Source: CAD feature listing. Evaluate the final solid. Frame: model axes, mm. Coordinates: 2 decimals unless noted, no trailing zeros. Order: outer loops, then holes, each group sorted by start corner. A loop starts at its lowest first (then second) coordinate and runs counter-clockwise, first axis right, second up.
```python
from build123d import *

# Parameters (mm, degrees)
BOSS_EXTRUDE3_DEPTH      = 2.4
BOSS_EXTRUDE3_DEPTH_BACK = 1.7
SKETCH5_W                = 0.3
SKETCH5_H                = 0.64
BOSS_EXTRUDE4_DEPTH      = 15


with BuildPart() as part:
    # Sketch4 → Boss-Extrude3 (new, two sides: drawn at the far end of the back side and taken through both)
    with BuildSketch(Plane(origin=(0, 0, 0), x_dir=(1, 0, 0), z_dir=(0, 1, 0)).offset(-BOSS_EXTRUDE3_DEPTH_BACK)):
        Polygon((0.8, 2.05), (1.6, 1.25), (1.6, -1.25), (0.8, -2.05), (0, -2.05), (0, 2.05), align=None)
    extrude(amount=BOSS_EXTRUDE3_DEPTH + BOSS_EXTRUDE3_DEPTH_BACK)

    # Sketch5 → Boss-Extrude4 (add)
    with BuildSketch(Plane.XZ.offset(1.7)):
        with Locations((0.65, 1.3)):
            Rectangle(SKETCH5_W, SKETCH5_H)
        with Locations((0.65, 0)):
            Rectangle(SKETCH5_W, SKETCH5_H)
        with Locations((0.65, -1.3)):
            Rectangle(SKETCH5_W, SKETCH5_H)
    extrude(amount=BOSS_EXTRUDE4_DEPTH)


solid = part.part
```
1. Section query B-B, the plane z = -0.05. Output: boundary loops of the cut face in (x, y).
2. Section query A-A, the plane y = -13.5. Output: boundary loops of the cut face in (x, z), plus the area to 3 significant figures.
3. Material intervals for line 1 along Z through (x, y) = (0.55, -3.5); line 2 along Y through (x, z) = (0.4, 0.05); line 3 along X through (y, z) = (-10.25, 1.2), sorted ascending.
4. Contact query for flat-ended pins moving along their axis: P1, Ø0.5, axis at y = -11, z = -1, coming from the -X side; P2, Ø0.5, axis at y = -9.5, z = 0, coming from the +X side; P3, Ø0.8, axis at x = 1, z = 0.5, coming from the -Y side. Output: stop coordinate, or through.
5. Section query C-C, the plane x = 1.05. Output: boundary loops of the cut face in (y, z).
6. Section query D-D, the plane z = 0.75. Output: boundary loops of the cut face in (x, y), plus the area to 3 significant figures.
Answer key:
1. outline: (0, -1.7) - (0.5, -1.7) - (0.5, -16.7) - (0.8, -16.7) - (0.8, -1.7) - (1.6, -1.7) - (1.6, 2.4) - (0, 2.4) - close
2. outline: (0.5, -1.62) - (0.8, -1.62) - (0.8, -0.98) - (0.5, -0.98) - close; (0.5, -0.32) - (0.8, -0.32) - (0.8, 0.32) - (0.5, 0.32) - close; (0.5, 0.98) - (0.8, 0.98) - (0.8, 1.62) - (0.5, 1.62) - close
2. area: 0.576 mm2
3. line 1: z = -1.62 to -0.98, -0.32 to 0.32, 0.98 to 1.62
3. line 2: y = -1.7 to 2.4
3. line 3: x = 0.5 to 0.8
4. P1: stops at x = 0.5
4. P2: stops at x = 0.8
4. P3: stops at y = -16.7
5. outline: (-1.7, -1.8) - (2.4, -1.8) - (2.4, 1.8) - (-1.7, 1.8) - close
6. outline: (0, -1.7) - (1.6, -1.7) - (1.6, 2.4) - (0, 2.4) - close
6. area: 6.56 mm2
